Part model, mm, in its own coordinate system. Face numbers are marked on the shaded views. A direction names the side the tool comes from. Round coordinates to 2 decimals unless told otherwise and drop trailing zeros. Write each loop counter-clockwise with the first axis right and the second up, starting at its lowest first coordinate (ties: lowest second). Pieces come first, ordered by that corner, then holes. Notation, with made-up numbers: M 27.25,36 L 62.25,36 A21 ccw 62.25,54 Z; hole C 14,-11.5 d9. An arc over 180 degrees is marked long. Use a Markdown table: item, result. Add a question column.
1) Slice it at D-D on z = 8.25. Write the cut outline in (x, y), plus the area to 3 significant figures.
2) Which spindle directions (+Z, -Z, +X, -X, +Y, -Y) get a long thin tool onto all of the face, cutting with end or side? Do the marked faces 1 and 2. Say none if no direction does.
3) Wall check: probe 1 along Y at (x, z) = (-4, 0.5); probe 2 along Y at (x, z) = (5.25, -7.5); probe 3 along X at (y, z) = (0.5, -9.25). Give the ranges that are in metal, low to high.
4) Slice it at C-C on z = -8.5. Write the cut outline in (x, y).
5) Drop flat-ended pins along their axis: P1, Ø6, axis at x = -5, z = 4, coming from the -Y side; P2, Ø0.5, axis at y = -6, z = -10, coming from the -X side; P3, Ø3, axis at x = -6.5, y = 26, coming from the -Z side; P4, Ø0.5, axis at x = 5, y = -2.5, coming from the +Z side. Give the stop position or say it passes through.
6) Slice it at B-B on y = 40.5. Write the cut outline in (x, z) (3 decimals).
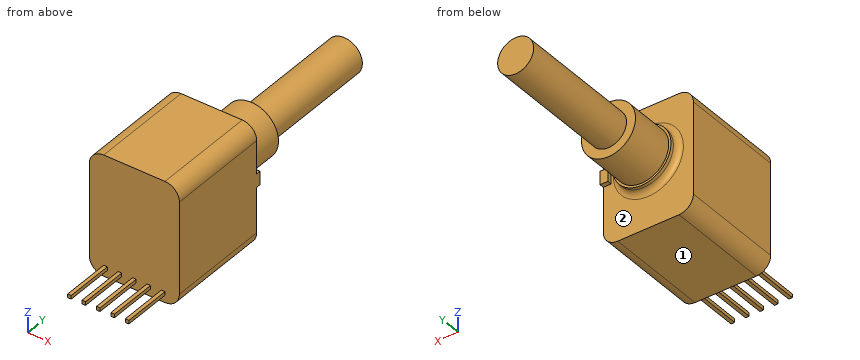
```python
from build123d import *

# Parameters (mm, degrees)
SKETCH1_W               = 15.875
SKETCH1_H               = 21.21
BODY_DEPTH              = 18.5
SKETCH2_R               = 4.7625
EXTRUDE_3_8_32_DEPTH    = 9.53
SKETCH4_R               = 3.175
SHAFT_DEPTH             = 22.225
SKETCH5_R               = 5.15874
BOSS_DEPTH              = 1.5875
SKETCH6_W               = 1.3716
SKETCH6_H               = 2.36
ANTI_ROTATION_LUG_DEPTH = 0.7874
SKETCH7_W               = 0.635
SKETCH7_H               = 0.635
PINS_DEPTH              = 8.636
FILLET1_R               = 1.016
FILLET2_R               = 2.54


with BuildPart() as part:
    # Sketch1 → body (new body)
    with BuildSketch(Plane(origin=(0, 0, 0), x_dir=(1, 0, 0), z_dir=(0, 1, 0))):
        with Locations((0, 1.08)):
            Rectangle(SKETCH1_W, SKETCH1_H)
    extrude(amount=BODY_DEPTH)

    # Sketch2 → 3/8-32 (add)
    with BuildSketch(Plane(origin=(0, 18.5, 0), x_dir=(1, 0, 0), z_dir=(0, 1, 0))):
        Circle(SKETCH2_R)
    extrude(amount=EXTRUDE_3_8_32_DEPTH)

    # Sketch4 → shaft (add)
    with BuildSketch(Plane(origin=(0, 28.03, 0), x_dir=(1, 0, 0), z_dir=(0, 1, 0))):
        Circle(SKETCH4_R)
    extrude(amount=SHAFT_DEPTH)

    # Sketch5 → boss (add)
    with BuildSketch(Plane(origin=(0, 18.5, 0), x_dir=(1, 0, 0), z_dir=(0, 1, 0))):
        Circle(SKETCH5_R)
    extrude(amount=BOSS_DEPTH)

    # Sketch6 → anti-rotation lug (add)
    with BuildSketch(Plane(origin=(0, 18.5, 0), x_dir=(1, 0, 0), z_dir=(0, 1, 0))):
        with Locations((7.2517, 0)):
            Rectangle(SKETCH6_W, SKETCH6_H)
    extrude(amount=ANTI_ROTATION_LUG_DEPTH)

    # Sketch7 → pins (add)
    with BuildSketch(Plane.XZ):
        with Locations((-5.08, -10.0975)):
            Rectangle(SKETCH7_W, SKETCH7_H)
        with Locations((-2.54, -10.0975)):
            Rectangle(SKETCH7_W, SKETCH7_H)
        with Locations((0, -10.0975)):
            Rectangle(SKETCH7_W, SKETCH7_H)
        with Locations((2.54, -10.0975)):
            Rectangle(SKETCH7_W, SKETCH7_H)
        with Locations((5.08, -10.0975)):
            Rectangle(SKETCH7_W, SKETCH7_H)
    extrude(amount=PINS_DEPTH)

    # Fillet1
    fillet1_edges = [part.edges().sort_by_distance(p)[0] for p in [
        (-5.15874, 18.5, 0),
    ]]
    fillet(fillet1_edges, radius=FILLET1_R)

    # Fillet2
    fillet2_edges = [part.edges().sort_by_distance(p)[0] for p in [
        (7.9375, 9.25, 9.525),
        (-7.9375, 9.25, 9.525),
        (-7.9375, 9.25, -11.685),
        (7.9375, 9.25, -11.685),
    ]]
    fillet(fillet2_edges, radius=FILLET2_R)


solid = part.part
```
Entries:
| question | item | result |
|---|---|---|
| 1 | outline | M -7.6,0 L 7.6,0 L 7.6,18.5 L -7.6,18.5 Z |
| 1 | area | 281 mm^2 |
| 2 | face 1 | -Z, +X, -X, +Y, -Y |
| 2 | face 2 | +Y |
| 3 | probe 1 | y = 0 to 28.03 |
| 3 | probe 2 | y = 0 to 18.5 |
| 3 | probe 3 | x = -7.94 to 7.94 |
| 4 | outline | M -7.94,0 L 7.94,0 L 7.94,18.5 L -7.94,18.5 Z |
| 5 | P1 | stops at y = 0 |
| 5 | P2 | stops at x = -5.4 |
| 5 | P3 | passes through |
| 5 | P4 | stops at z = -9.78 |
| 6 | outline | C 0,0 d6.35 |
